Could you check a few things on this model? Use its own coordinates, in mm. Face numbers are marked on the shaded views. Give positions to 0.01 mm unless a question says otherwise; leave off trailing zeros. Loops run counter-clockwise (first coordinate to the right, second up) from the corner with the lowest first, then second, coordinate; pieces in that order, holes last. Notation, with made-up numbers: (83, 68.25) - (128, 68.25) arc R25 ccw to (128, 99.25) - close; hole circle Ø2 at (60.5, 39.25). An arc over 180 degrees is marked (long way). Write each question's results on one line, items separated by ' | '. Start each with the question number.
(1) Suppose I cut it at D-D (y = -11). Please give me the cut outline in (x, z).
(2) Suppose I cut it at A-A (z = 0). Please give me the cut outline in (x, y).
(3) I need wall thicknesses on line 1 (X direction, y = 2, z = 0); line 2 (Z direction, x = 11, y = -14.5); line 3 (Z direction, x = -16, y = -16). Which ranges of each line are inside material? Lowest first, please.
(4) For pin 1 (1 mm diameter, centred on x = 6.5, z = 32, fed in from -Y); pin 2 (1 mm diameter, centred on x = 4, y = 2, fed in from +Z); pin 3 (5 mm diameter, centred on y = -9, z = -22.5, fed in from +X), each with a flat end and sliding along its axis, tell me the tip position at first contact or that it passes through.
(5) Suppose I cut it at C-C (y = -0.5). Please give me the cut outline in (x, z), and give its area (3 significant figures).
(6) Suppose I cut it at B-B (x = 0). Please give me the cut outline in (y, z), and give its area (3 significant figures).
(7) If we mould it in two halves opening along X, with no side actions, what happens to the marked faces 1 and 2? For each: released by +X, released by -X, zero draft, split by the parting line, or undercut.
from build123d import *


with BuildPart() as part:
    # Çizim1 → Döndür1 (revolve)
    with BuildSketch(Plane.XY, mode=Mode.PRIVATE) as d_nd_r1_sk:
        with BuildLine():
            Line((-25.1, 9.270415491), (-25.1, -4.129584509))
            ThreePointArc((-25.1, -4.129584509), (-30.067468991, -16.122115518), (-42.06, -21.089584509))
            Line((-42.06, -21.089584509), (-42.65, -21.089584509))
            Line((-42.65, -21.089584509), (-42.65, -20.339584509))
            Line((-42.65, -20.339584509), (-42.06, -20.339584509))
            Line((-42.06, -20.339584509), (-41.65, -20.339584509))
            Line((-41.65, -20.339584509), (-41.65, -19.584146943))
            ThreePointArc((-41.65, -19.584146943), (-30.984120802, -14.915524431), (-26.6, -4.129584509))
            Line((-26.6, -4.129584509), (-26.6, 9.270415491))
            Line((-26.6, 9.270415491), (-25.1, 9.270415491))
        make_face()
    revolve(d_nd_r1_sk.sketch.rotate(Axis((0, 0, 0), (0, 1, 0)), 270), axis=Axis((0, 0, 0), (0, 1, 0)))


solid = part.part
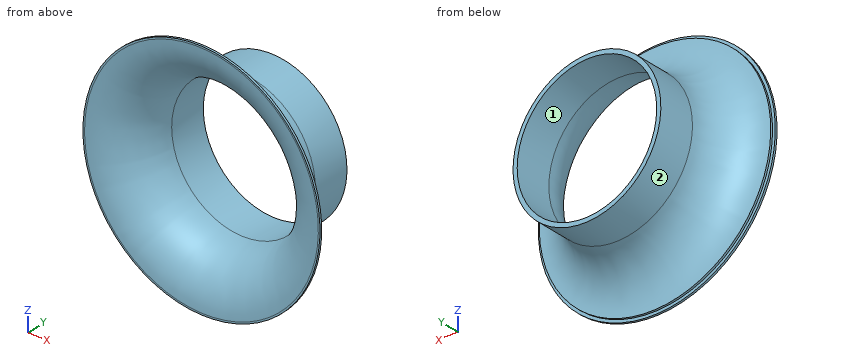
Output values:
1) outline: circle Ø56.42 at (0, 0); hole circle Ø53.11 at (0, 0)
2) outline: (-42.65, -21.09) - (-42.06, -21.09) arc R16.96 ccw to (-25.1, -4.13) - (-25.1, 9.27) - (-26.6, 9.27) - (-26.6, -4.13) arc R15.46 cw to (-41.65, -19.58) - (-41.65, -20.34) - (-42.65, -20.34) - close; (25.1, -4.13) arc R16.96 ccw to (42.06, -21.09) - (42.65, -21.09) - (42.65, -20.34) - (41.65, -20.34) - (41.65, -19.58) arc R15.46 cw to (26.6, -4.13) - (26.6, 9.27) - (25.1, 9.27) - close
3) line 1: -26.6 to -25.1, 25.1 to 26.6 | line 2: -28.55 to -26.44, 26.44 to 28.55 | line 3: -27.89 to -25.31, 25.31 to 27.89
4) pin 1: y = -18.56 | pin 2: z = 26.37 | pin 3: x = 19.05
5) outline: circle Ø53.2 at (0, 0); hole circle Ø50.2 at (0, 0) | area: 244 mm2
6) outline: (-21.09, -42.65) - (-20.34, -42.65) - (-20.34, -41.65) - (-19.58, -41.65) arc R15.46 cw to (-4.13, -26.6) - (9.27, -26.6) - (9.27, -25.1) - (-4.13, -25.1) arc R16.96 ccw to (-21.09, -42.06) - close; (-21.09, 42.06) arc R16.96 ccw to (-4.13, 25.1) - (9.27, 25.1) - (9.27, 26.6) - (-4.13, 26.6) arc R15.46 cw to (-19.58, 41.65) - (-20.34, 41.65) - (-20.34, 42.65) - (-21.09, 42.65) - close | area: 117 mm2
7) face 1: undercut | face 2: split by the parting line
